```python
from build123d import *

# Parameters (mm, degrees)
BOSS_EXTRUDE1_DEPTH = 1.5875
SCALE1_SCALE        = 0.8


with BuildPart() as part:
    # Sketch1 → Boss-Extrude1 (new body, symmetric)
    with BuildSketch(Plane.XY):
        with BuildLine():
            Line((-213.499711216, 186.497468723), (53.01875396, 492.542625266))
            ThreePointArc((53.01875396, 492.542625266), (92.447986648, 509.676487347), (130.603493871, 489.867628503))
            Line((130.603493871, 489.867628503), (243.695621782, 340.341208487))
            ThreePointArc((243.695621782, 340.341208487), (253.7875264, 308.456864193), (241.52355595, 277.343314433))
            Line((241.52355595, 277.343314433), (0, 0))
            ThreePointArc((0, 0), (-16.991876757, -12.670819234), (-37.70633704, -17.163554592))
            Line((-37.70633704, -17.163554592), (-82.399555371, -17.163554592))
            ThreePointArc((-82.399555371, -17.163554592), (-104.434529771, -12.046289615), (-121.959152061, 2.25804928))
            Line((-121.959152061, 2.25804928), (-215.352970866, 123.082627187))
            ThreePointArc((-215.352970866, 123.082627187), (-225.772036229, 155.121618903), (-213.499711216, 186.497468723))
        make_face()
    extrude(amount=BOSS_EXTRUDE1_DEPTH, both=True)


with BuildPart() as part_1:
    # Scale1: scaled about (0, 0, 0)
    add(part.part.scale(SCALE1_SCALE))


solid = part_1.part
```
Work out the finished part from the listing and answer in its coordinate system (mm). Coordinates: 2 decimals unless noted, no trailing zeros. Loops run counter-clockwise (first coordinate to the right, second up) from the corner with the lowest first, then second, coordinate; pieces in that order, holes last. Notation, with made-up numbers: (68.5, -4) - (114.5, -4) arc R17 cw to (114.5, 14) - close; hole circle Ø8 at (-20, 60.5). An arc over 180 degrees is marked (long way). Use a Markdown table: item, result.
Item 1: Find section A-A, the plane z = 0.8. Determine the outline of the cut face in (x, y) (1 decimal).
Evaluation:
| item | result |
|---|---|
| outline | (-172.3, 98.5) - (-97.6, 1.8) arc R40 ccw to (-65.9, -13.7) - (-30.2, -13.7) arc R40 ccw to (0, 0) - (193.2, 221.9) arc R40 ccw to (195, 272.3) - (104.5, 391.9) arc R40 ccw to (42.4, 394) - (-170.8, 149.2) arc R40 ccw to start |
Item 2: Find section B-B, the plane x = 37. Determine the outline of the cut face in (y, z).
Evaluation:
| item | result |
|---|---|
| outline | (42.49, -1.27) - (387.82, -1.27) - (387.82, 1.27) - (42.49, 1.27) - close |
Item 3: Given pin 1 Ø1.5 at (y, z) = (221, -1) entering from +X, flat-ended and moving along its own axis, determine where the tip first touches the part or whether it passes through.
Evaluation:
| item | result |
|---|---|
| pin 1 | stops at x = 193.11 |
Item 4: Find section C-C, the plane y = 254. Determine the outline of the cut face in (x, z), and give its area (3 significant figures).
Evaluation:
| item | result |
|---|---|
| outline | (-79.53, -1.27) - (202.62, -1.27) - (202.62, 1.27) - (-79.53, 1.27) - close |
| area | 717 mm2 |
Item 5: Consider probe 1 along X at (y, z) = (315, 0.1); probe 2 along X at (y, z) = (305, 0.65); probe 3 along Y at (x, z) = (175, 0.4). Determine where each line is inside the solid, lowest interval first. Write a range as from..to.
Evaluation:
| item | result |
|---|---|
| probe 1 | x = -26.41..162.64 |
| probe 2 | x = -35.12..170.2 |
| probe 3 | y = 200.95..298.66 |
